Here's the drawing with two shaded views (mm, measured from the low corner). I have some questions. A direction names the side the tool comes from. Coordinates: 2 decimals unless noted, no trailing zeros. Write each loop counter-clockwise with the first axis right and the second up, starting at its lowest first coordinate (ties: lowest second). Pieces come first, ordered by that corner, then holes. Notation, with made-up numbers: (-17.5, 81) -> (7.5, 81) arc R30 ccw to (7.5, 118) -> close; hole circle Ø9 at (21, -27). An arc over 180 degrees is marked (long way). Use one line per item in the form item = value.
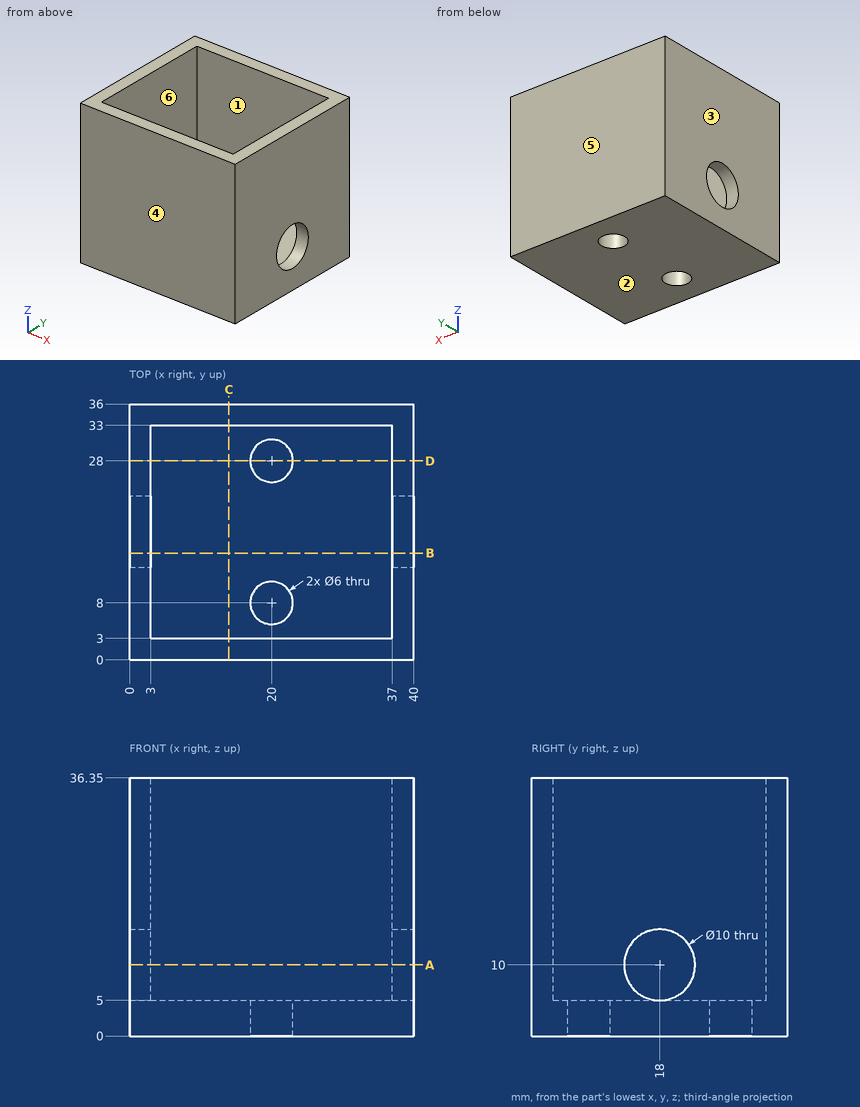
Q1. Suppose I cut it at D-D (y = 28). Write out the boundary of the cut face in (x, z), then the cut area to 3 significant figures.
Return value:
outline = (0, 0) -> (17, 0) -> (17, 5) -> (3, 5) -> (3, 36.35) -> (0, 36.35) -> close; (23, 0) -> (40, 0) -> (40, 36.35) -> (37, 36.35) -> (37, 5) -> (23, 5) -> close
area = 358 mm2
Q2. Suppose I cut it at A-A (z = 10). Write out the boundary of the cut face in (x, y), then the cut area to 3 significant figures.
Return value:
outline = (0, 0) -> (40, 0) -> (40, 13) -> (37, 13) -> (37, 3) -> (3, 3) -> (3, 13) -> (0, 13) -> close; (0, 23) -> (3, 23) -> (3, 33) -> (37, 33) -> (37, 23) -> (40, 23) -> (40, 36) -> (0, 36) -> close
area = 360 mm2
Q3. Suppose I cut it at C-C (x = 14). Write out the boundary of the cut face in (y, z).
Return value:
outline = (0, 0) -> (36, 0) -> (36, 36.35) -> (33, 36.35) -> (33, 5) -> (3, 5) -> (3, 36.35) -> (0, 36.35) -> close
Q4. Suppose I cut it at B-B (y = 15). Write out the boundary of the cut face in (x, z).
Return value:
outline = (0, 0) -> (40, 0) -> (40, 6) -> (37, 6) -> (37, 5) -> (3, 5) -> (3, 6) -> (0, 6) -> close; (0, 14) -> (3, 14) -> (3, 36.35) -> (0, 36.35) -> close; (37, 14) -> (40, 14) -> (40, 36.35) -> (37, 36.35) -> close
Q5. If I drill on line 1 (Y direction, x = 20, z = 3); line 2 (Z direction, x = 0.7, y = 18); line 3 (Y direction, x = 2.25, z = 10), over which ranges is the centre line in solid material (lowest first)? Write a range as from..to.
Return value:
line_1 = 0..5, 11..25, 31..36
line_2 = 0..5, 15..36.35
line_3 = 0..13, 23..36
Q6. For the marked faces 1 and 2, which set-ups out of +Z, -Z, +X, -X, +Y, -Y let a thin tool reach every point of the face, with its end or its side?
Return value:
face_1 = +Z
face_2 = -Z, +X, -X, +Y, -Y
Q7. Will these pins go through, and if not, where does the flat tip stop? pin 1 (5 mm diameter, centred on x = 5.5, y = 16, fed in from -Z); pin 2 (6 mm diameter, centred on x = 17.5, y = 24, fed in from +Z).
Return value:
pin_1 = 0
pin_2 = 5
Q8. Thinking about a two-plate mould opening in Y: for the marked faces 3, 4, 5 and 6, which applies, released by +Y, released by -Y, zero draft, split by the parting line, or undercut?
Return value:
face_3 = zero draft
face_4 = released by -Y
face_5 = released by +Y
face_6 = undercut
